Autodesk Inventor part; units mm, degrees
ref_plane "XY Plane" through (0, 0, 0) normal (0, 0, 1) x (1, 0, 0)
sketch "Sketch1" plane through (0, 0, 0) normal (0, 0, 1) x (1, 0, 0)
  line L0 (-19.5, 0) -> (19.5, 0) construction
  line L1 (-1.118, -1) -> (1.118, -1)
  line L2 (0, -3.5) -> (0, -10.5) construction
  line L3 (0, 31.6864) -> (0, -32.6182) construction
  line L4 (2, -2.8723) -> (2, -19.3972)
  line L5 (-2, -2.8723) -> (-2, -19.3972)
  line L6 (3.0311, 1.75) -> (9.0933, 5.25) construction
  line L7 (-3.0311, 1.75) -> (-9.0933, 5.25) construction
  line L8 (3.4875, -0.2959) -> (17.7984, 7.9665)
  line L9 (1.4875, 3.1682) -> (15.7984, 11.4306)
  arc A0 (2, -19.3972) -> (17.7984, 7.9665) centre (0, 0) ccw
  line L10 (-15.7984, 11.4306) -> (-1.4875, 3.1682)
  line L11 (-17.7984, 7.9665) -> (-3.4875, -0.2959)
  arc A1 (15.7984, 11.4306) -> (-15.7984, 11.4306) centre (0, 0) ccw
  arc A2 (-17.7984, 7.9665) -> (-2, -19.3972) centre (0, 0) ccw
  arc A3 (-3.4875, -0.2959) -> (-2, -2.8723) centre (0, 0) ccw
  arc A4 (2, -2.8723) -> (3.4875, -0.2959) centre (0, 0) ccw
  line L12 (0, 0) -> (2.0417, 7.6198) construction
  line L13 (0, 0) -> (-1.8775, 7.0067) construction
  line L14 (0.3882, 1.4489) -> (0.9059, 3.3807)
  line L15 (-0.3882, 1.4489) -> (-0.9059, 3.3807)
  arc A5 (1.4875, 3.1682) -> (0.9059, 3.3807) centre (0, 0) ccw
  arc A6 (-0.9059, 3.3807) -> (-1.4875, 3.1682) centre (0, 0) ccw
  arc A7 (1.118, -1) -> (0.3882, 1.4489) centre (0, 0) ccw
  arc A8 (-0.3882, 1.4489) -> (-1.118, -1) centre (0, 0) ccw
  circle A9 centre (0, 0) radius 22.5
  dimension "d3" = 1
  dimension "d4" = 2
  dimension "d5" = 2
  dimension "d8" = 360
  dimension "d10" = 2
  dimension "d11" = 2
  dimension "d12" = 2
  dimension "d13" = 2
  dimension "d17" = 3.5
  dimension "d18" = 3.5
  dimension "d19" = 15
  dimension "d20" = 15
  dimension "d21" = 3.5
  dimension "d22" = 3.5
  dimension "d23" = 1.5
  dimension "d24" = 1.5
  dimension "d25" = 45
  dimension "d81" = 3
  dimension "d84" = 3
  dimension "d85" = 3
extrude "Extrusion1" add sketch "Sketch1" along normal blind 6
fillet "Fillet10" radius 1 6 edges at (3.4875, -0.2959, 3) (2, -2.8723, 3) (-3.4875, -0.2959, 3) (-2, -2.8723, 3) (-1.4875, 3.1682, 3) (1.4875, 3.1682, 3)
fillet "Fillet11" radius 3 6 edges at (-17.7984, 7.9665, 3) (-15.7984, 11.4306, 3) (15.7984, 11.4306, 3) (17.7984, 7.9665, 3) (2, -19.3972, 3) (-2, -19.3972, 3)
sketch "Sketch4" plane through (0, 0, 0) normal (0, 1, 0) x (-1, 0, 0)
  circle A0 centre (22.26, 3.2046) radius 1.5
  line L0 (0, 7.6708) -> (0, -6.5685) construction
  line L1 (22.4632, 5.9906) -> (22.4632, 0) construction
  point P0 (0, 0)
  dimension "d77" = 3
revolve "Revolution2" cut sketch "Sketch4" angle 360 about axis through (0, 0, 7.6708) along (0, 0, -1)
equation "\"d5\" = d4"
equation "\"d11\" = d10"
equation "\"d12\" = d10"
equation "\"d13\" = d10"
equation "\"d18\" = d17"
equation "\"d20\" = d19"
equation "\"d21\" = d17"
equation "\"d22\" = d17"
equation "\"d24\" = d23"
properties part number "Rueda1"
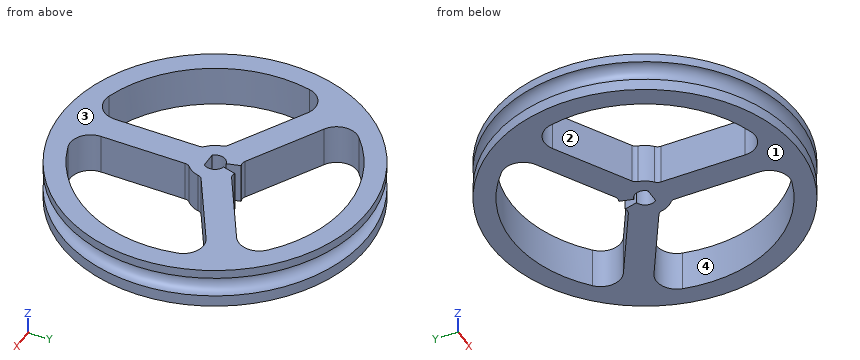
Input: part model. Units: mm. Frame: model coordinates. Face numbers are marked on the shaded views. A direction names the side the tool comes from. Give positions to 0.01 mm unless a question says otherwise; leave off trailing zeros. Put each result on its own line as item: value.
Item 1: Draft query along X for the marked faces 1 and 2. Return one class per face: +X half, -X half, draft (parallel to the pull), parting line (faces both ways), or undercut.
Found:
face 1: draft
face 2: undercut
Item 2: Access query for the marked faces 3 and 4. Directions: +Z, -Z, +X, -X, +Y, -Y. A direction counts if a zero-diameter tool reaches every point of the face in a straight line with its end or side. Return the directions, or none.
Found:
face 3: +Z, +X, -X, +Y, -Y
face 4: +Z, -Z
Item 3: Ray query, L1, parallel to X at y = -8, z = 5.1; L2, parallel to Y at x = -1, z = 5.25; L3, parallel to X at y = -11, z = 0.7. Return the intervals inside material, ascending. Write a range as from..to.
Found:
L1: x = -21.03..-17.78, -2..2, 17.78..21.03
L2: y = -22.48..-1, 1.12..3.35, 19.47..22.48
L3: x = -19.63..-16.1, -2..2, 16.1..19.63
Item 4: Contact query for flat-ended pins moving along their axis: pin 1 (2.5 mm diameter, centred on x = 0, z = 2.5, fed in from +Y); pin 2 (4 mm diameter, centred on x = -15.5, y = -7.5, fed in from -Z); pin 3 (3 mm diameter, centred on y = -9, z = 4.5, fed in from -X); pin 4 (3 mm diameter, centred on y = -12, z = 3.5, fed in from +X). Output: stop coordinate, or through.
Found:
pin 1: stops at y = 22.5
pin 2: passes through
pin 3: stops at x = -21.21
pin 4: stops at x = 19.58
Item 5: Section query A-A, the plane z = 2.45. Count the separate pieces of the cut face and the enclosed holes in it, then the cut area to 3 significant figures.
Found:
separate pieces: 1
enclosed holes: 3
area: 430 mm^2
